Autodesk Inventor part; units mm, degrees
ref_plane "YZ Plane" through (0, 0, 0) normal (1, 0, 0) x (0, 1, 0)
ref_plane "XZ Plane" through (0, 0, 0) normal (0, 1, 0) x (-1, 0, 0)
ref_plane "XY Plane" through (0, 0, 0) normal (0, 0, 1) x (1, 0, 0)
sketch "Sketch1" plane through (0, 0, 0) normal (1, 0, 0) x (0, 1, 0)
  line L0 (-8.5, -445) -> (-8.5, -5)
  line L1 (11.5, -5) -> (11.5, -445)
  line L2 (-8.5, -5) -> (-1.5, -5)
  line L3 (-1.5, -5) -> (-1.5, 2)
  line L4 (-1.5, 2) -> (-8.5, 2)
  line L5 (-8.5, 2) -> (-8.5, -5)
  line L6 (11.5, -5) -> (4.5, -5)
  line L7 (4.5, -5) -> (4.5, 2)
  line L8 (4.5, 2) -> (11.5, 2)
  line L9 (11.5, 2) -> (11.5, -5)
  line L10 (11.5, 8) -> (4.5, 8)
  line L11 (4.5, 8) -> (4.5, 15)
  line L12 (4.5, 15) -> (11.5, 15)
  line L13 (11.5, 15) -> (11.5, 8)
  line L14 (-8.5, 8) -> (-1.5, 8)
  line L15 (-1.5, 8) -> (-1.5, 15)
  line L16 (-1.5, 15) -> (-8.5, 15)
  line L17 (-8.5, 15) -> (-8.5, 8)
  line L18 (5.5, 1) -> (-2.5, 1)
  line L19 (-2.5, 1) -> (-2.5, 9)
  line L20 (-2.5, 9) -> (5.5, 9)
  line L21 (5.5, 9) -> (5.5, 1)
  point P0 (0, 0)
  point P1 (5.5, 2)
  point P2 (5.5, 8)
  point P3 (4.5, 9)
  point P4 (-1.5, 9)
  point P5 (-2.5, 8)
  point P6 (-2.5, 2)
  point P7 (-1.5, 1)
  point P8 (4.5, 1)
  dimension "d0" = 7
  dimension "d1" = 7
  dimension "d2" = 7
  dimension "d3" = 7
  dimension "d4" = 7
  dimension "d5" = 7
  dimension "d6" = 7
  dimension "d7" = 7
  dimension "d8" = 6
  dimension "d9" = 8
  dimension "d10" = 8
  dimension "d11" = 1
  dimension "d12" = 1
extrude "Extrusion1" add sketch "Sketch1" along normal blind 162 and the other way blind 18
properties part number "ybar"
Build history of the part. All positions in model axes, mm. A direction names the side the tool comes from. Round coordinates to 2 decimals unless told otherwise and drop trailing zeros. Write each loop counter-clockwise with the first axis right and the second up, starting at its lowest first coordinate (ties: lowest second). Pieces come first, ordered by that corner, then holes. Notation, with made-up numbers: M 87.25,41 L 106.25,41 A24 ccw 106.25,63 Z; hole C 0,42.5 d8. An arc over 180 degrees is marked long. Answer as a JSON object with one key per item and string values. Group by question number.
(1) Cut at D-D (z = 6.5). Give the cut face in (x, y), and give its area (3 significant figures).
(2) Drill centre lines: L1, parallel to Z at x = 35.5, y = -6.5; L2, parallel to Y at x = 127.5, z = 14.25; L3, parallel to Z at x = 122, y = 2. Where is each one in solid material? Low to high.
(3) Cut at A-A (y = -5.25). Give the cut face in (x, z).
(4) Mould opens along Y. For faces 1 (the flat face through (71, 11.5, 12)), 2 (the flat face through (71, -1.5, 12)), 3 (the flat face through (71, -8.5, -1)) say: pulls with the +Y half, pulls with the -Y half, needs draft (parallel to the pull), parting line crosses it, or undercut.
(5) Flat gauge pins, fed straight in: pin 1 (1.5 mm diameter, centred on x = 89.5, z = 6.5, fed in from -Y); pin 2 (1.5 mm diameter, centred on y = 3.5, z = 10, fed in from +X); pin 3 (1.8 mm diameter, centred on x = 60.5, z = 4.5, fed in from +Y). Where does each tip first touch, or does it go through?
(6) Which spindle directions (+Z, -Z, +X, -X, +Y, -Y) get a long thin tool onto all of the face, cutting with end or side? Do faces 4 (the flat face through (71, 9, 8)), 5 (the flat face through (71, -2.5, 5)), 6 (the flat face through (71, 2, 1)), 7 (the flat face through (71, 1, 9)), 8 (the flat face through (71, -5, 15)). Say none if no direction does.
(7) Cut at C-C (x = 57.5). Give the cut face in (y, z).
(8) Cut at B-B (z = -3.5). Give the cut face in (x, y), and give its area (3 significant figures).
Responses:
{
 "1": {"outline": "M -18,-2.5 L 162,-2.5 L 162,5.5 L -18,5.5 Z", "area": "1,440 mm2"},
 "2": {"L1": "z = -5 to 2, 8 to 15", "L2": "y = -8.5 to -1.5, 4.5 to 11.5", "L3": "z = 1 to 9"},
 "3": {"outline": "M -18,-5 L 162,-5 L 162,2 L -18,2 Z; M -18,8 L 162,8 L 162,15 L -18,15 Z"},
 "4": {"face 1": "pulls with the +Y half", "face 2": "undercut", "face 3": "pulls with the -Y half"},
 "5": {"pin 1": "stops at y = -2.5", "pin 2": "passes through", "pin 3": "stops at y = 5.5"},
 "6": {"face 4": "+X, -X, +Y", "face 5": "+X, -X, -Y", "face 6": "-Z, +X, -X", "face 7": "+Z, +X, -X", "face 8": "+Z, +X, -X, +Y, -Y"},
 "7": {"outline": "M -8.5,-5 L -1.5,-5 L -1.5,1 L 4.5,1 L 4.5,-5 L 11.5,-5 L 11.5,2 L 5.5,2 L 5.5,8 L 11.5,8 L 11.5,15 L 4.5,15 L 4.5,9 L -1.5,9 L -1.5,15 L -8.5,15 L -8.5,8 L -2.5,8 L -2.5,2 L -8.5,2 Z"},
 "8": {"outline": "M -18,-8.5 L 162,-8.5 L 162,-1.5 L -18,-1.5 Z; M -18,4.5 L 162,4.5 L 162,11.5 L -18,11.5 Z", "area": "2,520 mm2"}
}
